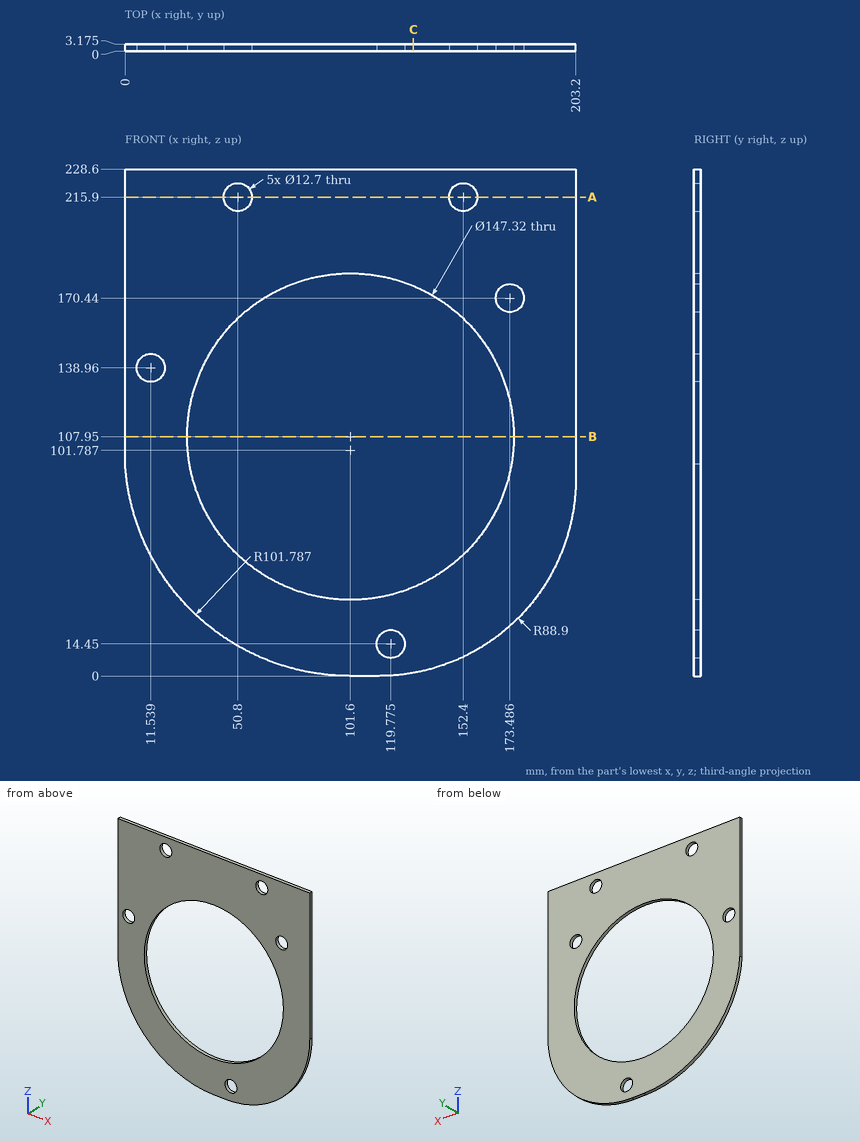
The figure shows three views and two pictorial views of one solid part (mm, origin at its lowest corner). Answer the questions. Give positions to 0.01 mm unless a question says otherwise; leave off trailing zeros. Order: outer loops, then holes, each group sorted by start corner. A loop starts at its lowest first (then second) coordinate and runs counter-clockwise, first axis right, second up. Notation, with made-up numbers: M 0,45 L 32,45 A19 cw 32,58 Z; hole C -33.5,29 d1. An arc over 180 degrees is marked long. Return JSON: item names as keys, results as strings.
Q1. Find section B-B, the plane z = 107.95. Write down the section's boundary in (x, y) (1 decimal).
Answer below:
{"outline": "M 0,0 L 27.9,0 L 27.9,3.2 L 0,3.2 Z; M 175.3,0 L 203.2,0 L 203.2,3.2 L 175.3,3.2 Z"}
Q2. This flat-tipped pin is pushed along its axis until it touches: pin 1 (1.5 mm diameter, centred on y = 0.5, z = 25.5, fed in from -X) (1 decimal). Where does it stop, or does it pass through?
Answer below:
{"pin 1": "stops at x = 33.4"}
Q3. Find section A-A, the plane z = 215.9. State how many separate pieces and enclosed holes the cut face has.
Answer below:
{"separate pieces": "3", "enclosed holes": "0"}
Q4. Find the intervals of material crossed by line 1 along X through (y, z) = (1.9, 107.95); line 2 along Z through (x, y) = (150, 0.8) (1 decimal); line 3 along Z through (x, y) = (54.5, 1.85) (1 decimal), in increasing order. Write a range as [from, to].
Answer below:
{"line 1": "x = [0, 27.94], [175.26, 203.2]", "line 2": "z = [7.5, 52.4], [163.5, 210], [221.8, 228.6]", "line 3": "z = [11.6, 51.3], [164.6, 210.7], [221.1, 228.6]"}
Q5. Find section C-C, the plane x = 130. Write down the section's boundary in (y, z) (1 decimal).
Answer below:
{"outline": "M 0,1.4 L 3.2,1.4 L 3.2,40 L 0,40 Z; M 0,175.9 L 3.2,175.9 L 3.2,228.6 L 0,228.6 Z"}
